from build123d import *

# Parameters (mm, degrees)
F0_W     = 20
F0_H     = 30
F1_DEPTH = 2
F3_DEPTH = 11
F4_R     = 2
F5_DEPTH = 25
F6_R     = 1
F7_R     = 2.230975


with BuildPart() as f1:
    # F0 (on Top) → F1 (new body)
    with BuildSketch(Plane.XY):
        Rectangle(F0_W, F0_H)
        Polygon((-4, 11.862541), (0, 10), (4, 11.862541), (4, -10), (-4, -10), align=None, mode=Mode.SUBTRACT)
    extrude(amount=F1_DEPTH)

    # F2 (on face) → F3 (join)
    with BuildSketch(Plane.XY.offset(2)):
        Polygon((-2.2, 10), (0, 10), (2.2, 10), (5.155044, 13), (8, 13), (8, -15), (10, -15), (10, 15), (-10, 15), (-10, -15), (-8, -15), (-8, 13), (-5.155044, 13), align=None)
    extrude(amount=F3_DEPTH)

    # F4 (on face) → F5 (join)
    with BuildSketch(Plane.XZ.offset(-10)):
        with Locations((0, 10.5)):
            Circle(F4_R)
    extrude(amount=F5_DEPTH)

    # F6
    f6_edges = [f1.edges().sort_by_distance(p)[0] for p in [
        (2.2, 10, 7.5),
        (-2.2, 10, 7.5),
    ]]
    fillet(f6_edges, radius=F6_R)

    # F7
    f7_edges = [f1.edges().sort_by_distance(p)[0] for p in [
        (0, 10, 1),
    ]]
    fillet(f7_edges, radius=F7_R)


with BuildPart() as f8_1:
    # F8: copy of F1
    add(f1.part.moved(Location((43.7, 0, 0))))


solid = f1.part
Verification items for the finished model (mm, model axes). A direction names the side the tool comes from. Coordinates: 2 decimals unless noted, no trailing zeros. Write each loop counter-clockwise with the first axis right and the second up, starting at its lowest first coordinate (ties: lowest second). Pieces come first, ordered by that corner, then holes. Notation, with made-up numbers: M 82.5,54 L 102.5,54 A6 ccw 102.5,65 Z; hole C 7,8 d11. An arc over 180 degrees is marked long. Use CSV: the item, a comma, the result in double quotes.
Q1. Section check A-A, the plane x = 0. Enter the section's corners in (y, z).
Computed values:
outline,"M -15,0 L -10,0 L -10,2 L -15,2 Z; M -15,8.5 L 10,8.5 L 10,2 L 10.23,2 L 10.23,0 L 15,0 L 15,13 L 10,13 L 10,12.5 L -15,12.5 Z"
Q2. Thickness scan on line 1 along X through (y, z) = (-4.5, 6.25); line 2 along X through (y, z) = (-8, 9.75); line 3 along Y through (x, z) = (7.25, 9.5). Record the ranges inside material, lowest first. Write a range as [from, to].
Computed values:
line 1,"[-10, -8], [8, 10]"
line 2,"[-10, -8], [-1.85, 1.85], [8, 10]"
line 3,"[13, 15]"
Q3. Section check B-B, the plane y = -11.5. Enter the section's corners in (x, z).
Computed values:
outline,"M -10,0 L 10,0 L 10,13 L 8,13 L 8,2 L -8,2 L -8,13 L -10,13 Z; C 0,10.5 d4"
Q4. Section check D-D, the plane y = -2. Enter the section's corners in (x, z), and give its area (3 significant figures).
Computed values:
outline,"M -10,0 L -4,0 L -4,2 L -8,2 L -8,13 L -10,13 Z; C 0,10.5 d4; M 4,0 L 10,0 L 10,13 L 8,13 L 8,2 L 4,2 Z"
area,"80.6 mm²"
Q5. Section check C-C, the plane z = 5.25. Enter the section's corners in (x, y).
Computed values:
outline,"M -10,-15 L -8,-15 L -8,13 L -5.16,13 L -2.49,10.3 A1 ccw -1.78,10 L 1.78,10 A1 ccw 2.49,10.3 L 5.16,13 L 8,13 L 8,-15 L 10,-15 L 10,15 L -10,15 Z"
Q6. Set-up check for faces 5 (the flat face through (-4, 1, 1)), 6 (the flat face through (2.45, 11.14, 0.99)), 7 (the flat face through (0, 10, 12.7)): record each of +Z, -Z, +X, -X, +Y, -Y from which the full face is reachable in a straight line by a thin tool's end or side.
Computed values:
face 5,"+Z, -Z"
face 6,"-Z"
face 7,"+Z, -Y"
Q7. Mould release check, pull along Y, two halves, no side actions. Record for faces 1 (the flat face through (0, 15, 6)), 2 (the cylindrical face through (-0.26, -2.325, 12.483)), 3 (the cylindrical face through (-0.01, 10.23, 1.01)), 4 (the flat face through (-2.49, 11.16, 0.99)): pulls with the +Y half, pulls with the -Y half, needs draft (parallel to the pull), parting line crosses it, or undercut.
Computed values:
face 1,"pulls with the +Y half"
face 2,"needs draft"
face 3,"undercut"
face 4,"undercut"
Q8. Go/stop test with flat-tipped pins: P1, Ø1.7, axis at x = -0.5, z = 12.5, coming from the -Y side; P2, Ø4, axis at x = 0.5, z = 5.5, coming from the -Y side; P3, Ø2.5, axis at x = -6, z = 9, coming from the -Y side; P4, Ø1.4, axis at x = 7, z = 6, coming from the -Y side. Record where each tip stops, or that it passes through.
Computed values:
P1,"y = -15"
P2,"y = 10"
P3,"y = 12.59"
P4,"y = 13"
